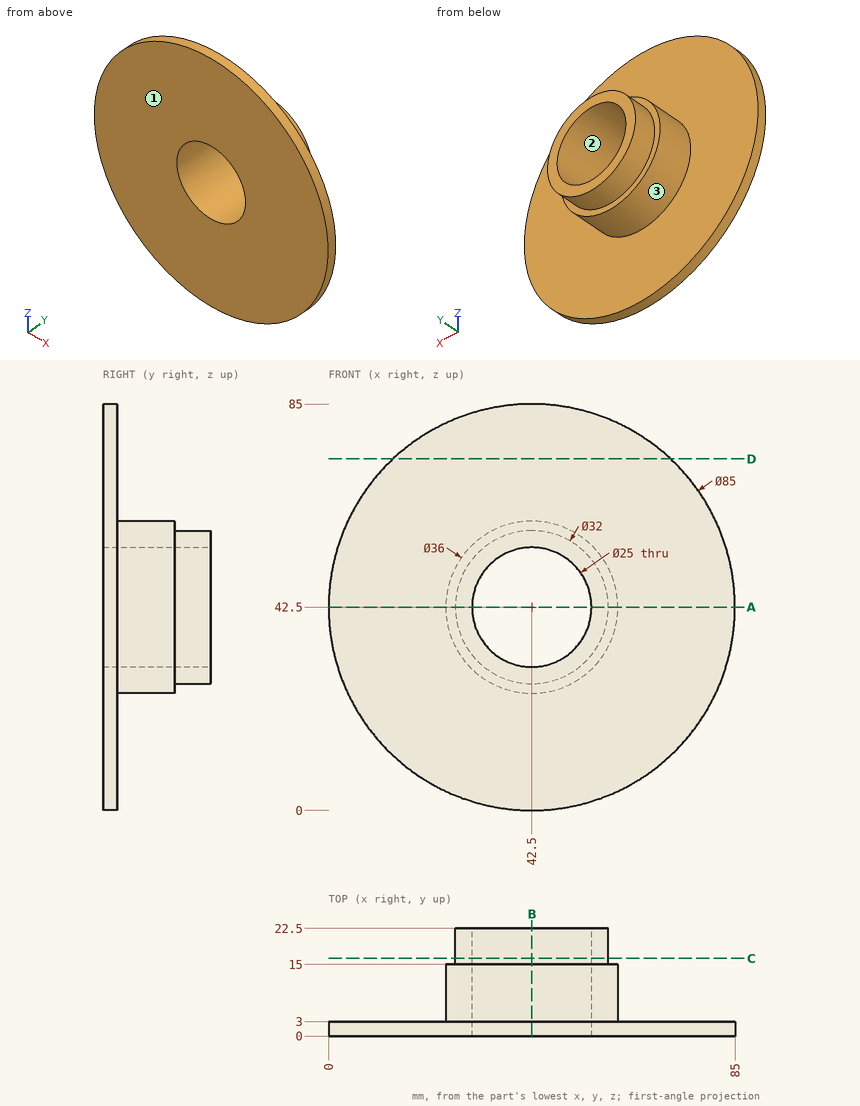
Print and shaded views of the part. All mm, measured from the part's lowest x, y and z. Round coordinates to 2 decimals unless told otherwise and drop trailing zeros. Write each loop counter-clockwise with the first axis right and the second up, starting at its lowest first coordinate (ties: lowest second). Pieces come first, ordered by that corner, then holes.
Item 1: Probe L1, parallel to X at y = 14.5, z = 42.5; L2, parallel to Y at x = 21, z = 73.5. List the from-to ranges inside material, lowest first.
Results:
L1: x = 24.5 to 30, 55 to 60.5
L2: y = 0 to 3
Item 2: Cut at B-B, the plane x = 42.5. Give the cut face in (y, z), plus the area to 4 significant figures.
Results:
outline: (0, 0) - (3, 0) - (3, 24.5) - (15, 24.5) - (15, 26.5) - (22.5, 26.5) - (22.5, 30) - (0, 30) - close; (0, 55) - (22.5, 55) - (22.5, 58.5) - (15, 58.5) - (15, 60.5) - (3, 60.5) - (3, 85) - (0, 85) - close
area: 364.5 mm2
Item 3: Drop flat-ended pins along their axis: pin 1 Ø1 at (y, z) = (11, 31.5) entering from +X; pin 2 Ø1.5 at (x, y) = (43.5, 11.5) entering from +Z; pin 3 Ø2 at (x, y) = (35, 6) entering from -Z. Give the stop position or say it passes through.
Results:
pin 1: stops at x = 57.12
pin 2: stops at z = 60.5
pin 3: stops at z = 25.71
Item 4: Cut at D-D, the plane z = 73.5. Give the cut face in (x, y), plus the area to 3 significant figures.
Results:
outline: (13.43, 0) - (71.57, 0) - (71.57, 3) - (13.43, 3) - close
area: 174 mm2
Item 5: Cut at A-A, the plane z = 42.5. Give the cut face in (x, y).
Results:
outline: (0, 0) - (30, 0) - (30, 22.5) - (26.5, 22.5) - (26.5, 15) - (24.5, 15) - (24.5, 3) - (0, 3) - close; (55, 0) - (85, 0) - (85, 3) - (60.5, 3) - (60.5, 15) - (58.5, 15) - (58.5, 22.5) - (55, 22.5) - close
Item 6: Cut at C-C, the plane y = 16.25. Give the cut face in (x, z).
Results:
outline: circle Ø32 at (42.5, 42.5); hole circle Ø25 at (42.5, 42.5)
Item 7: Two-plate mould, pull along Z, no slides. Class the marked faces 1, 2 and 3: +Z half, -Z half, draft (parallel to the pull), parting line (faces both ways), or undercut.
Results:
face 1: draft
face 2: undercut
face 3: parting line
